Build history of the part. All positions in model axes, mm. Face numbers are marked on the shaded views. Give positions to 0.01 mm unless a question says otherwise; leave off trailing zeros. Order: outer loops, then holes, each group sorted by start corner. A loop starts at its lowest first (then second) coordinate and runs counter-clockwise, first axis right, second up. Notation, with made-up numbers: (10.25, 27) -> (22.25, 27) arc R14 cw to (22.25, 40) -> close; hole circle Ø11 at (15.5, -17). An arc over 180 degrees is marked (long way). One line per item, written item: value. Start each with the question number.
(1) Probe line 1 (X direction, y = 40, z = -12); line 2 (X direction, y = -5, z = 1); line 3 (Y direction, x = -14.5, z = -2.5). List the from-to ranges inside material, lowest first.
(2) Saw through at A-A on x = 0. Give the cut face in (y, z) (3 decimals), plus the area to 3 significant figures.
(3) Saw through at D-D on z = -11. Give the cut face in (x, y).
(4) Saw through at B-B on y = 0. Give the cut face in (x, z) (3 decimals), plus the area to 3 significant figures.
(5) Pin check, flat tips, straight feed: pin 1 (3.5 mm diameter, centred on x = -25, y = -1.5, fed in from +Z) (3 decimals); pin 2 (3.5 mm diameter, centred on x = -15, z = 0, fed in from +Y); pin 3 (23 mm diameter, centred on x = 0, y = 0, fed in from +Z). Stop position of each tip, or through.
(6) Saw through at C-C on x = -30. Give the cut face in (y, z) (3 decimals).
(7) Two-plate mould, pull along Y, no slides. Class the marked faces 1, 2 and 3: +Y half, -Y half, draft (parallel to the pull), parting line (faces both ways), or undercut.
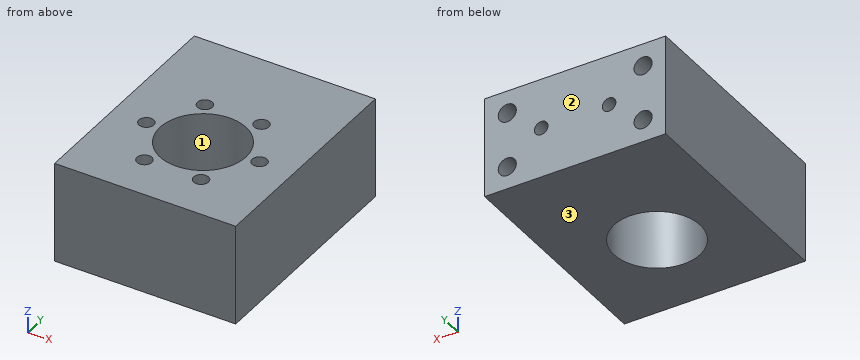
```python
from build123d import *

# Parameters (mm, degrees)
ESBO_O2_W                = 80
ESBO_O2_H                = 117.2
RESSALTO_EXTRUS_O2_DEPTH = 22.225
ESBO_O3_R                = 19
CORTE_EXTRUS_O1_DEPTH    = 45.45
ESBO_O4_R                = 3.3
CORTE_EXTRUS_O2_DEPTH    = 34.5
PADR_OCIRCULAR1_COUNT    = 6
ESBO_O10_R               = 4
ESBO_O10_R_2             = 3
CORTE_EXTRUS_O5_DEPTH    = 30
ESBO_O12_W               = 80
ESBO_O12_H               = 17.2
CORTE_EXTRUS_O7_DEPTH    = 45.45


with BuildPart() as part:
    # Esboço2 → Ressalto-extrusão2 (new body, symmetric)
    with BuildSketch(Plane.XY):
        Rectangle(ESBO_O2_W, ESBO_O2_H)
    extrude(amount=RESSALTO_EXTRUS_O2_DEPTH, both=True)

    # Esboço3 → Corte-extrusão1 (cut, through all)
    with BuildSketch(Plane.XY.offset(22.225)):
        Circle(ESBO_O3_R)
    extrude(amount=-CORTE_EXTRUS_O1_DEPTH, mode=Mode.SUBTRACT)

    # Esboço4 → Corte-extrusão2 (cut)
    with BuildSketch(Plane.XY.offset(22.225)):
        with Locations((12.5, 21.650635095)):
            Circle(ESBO_O4_R)
    corte_extrus_o2 = extrude(amount=-CORTE_EXTRUS_O2_DEPTH, mode=Mode.SUBTRACT)

    # PadrãoCircular1: Corte-extrusão2 ×6 about axis
    padr_ocircular1_axis = Axis((0, 0, 0), (0, 0, 1))
    for i in range(1, PADR_OCIRCULAR1_COUNT):
        add(corte_extrus_o2.rotate(padr_ocircular1_axis, i * 360 / PADR_OCIRCULAR1_COUNT), mode=Mode.SUBTRACT)

    # Esboço10 → Corte-extrusão5 (cut)
    with BuildSketch(Plane(origin=(0, 58.6, 0), x_dir=(1, 0, 0), z_dir=(0, 1, 0))):
        with Locations((-30, 12.225)):
            Circle(ESBO_O10_R)
        with Locations((30, 12.225)):
            Circle(ESBO_O10_R)
        with Locations((-30, -12.225)):
            Circle(ESBO_O10_R)
        with Locations((30, -12.225)):
            Circle(ESBO_O10_R)
        with Locations((-15, 0)):
            Circle(ESBO_O10_R_2)
        with Locations((15, 0)):
            Circle(ESBO_O10_R_2)
    extrude(amount=-CORTE_EXTRUS_O5_DEPTH, mode=Mode.SUBTRACT)

    # Esboço12 → Corte-extrusão7 (cut, through all)
    with BuildSketch(Plane.XY.offset(22.225)):
        with Locations((0, -50)):
            Rectangle(ESBO_O12_W, ESBO_O12_H)
    extrude(amount=-CORTE_EXTRUS_O7_DEPTH, mode=Mode.SUBTRACT)


solid = part.part
```
Results below:
1. line 1: x = -40 to -33.99, -26.01 to 26.01, 33.99 to 40
1. line 2: x = -40 to -18.33, 18.33 to 40
1. line 3: y = -41.4 to -24.28, -19.03 to -12.28, 12.28 to 19.03, 24.28 to 28.6
2. outline: (-41.4, -22.225) -> (-19, -22.225) -> (-19, 22.225) -> (-41.4, 22.225) -> close; (19, -22.225) -> (58.6, -22.225) -> (58.6, 22.225) -> (19, 22.225) -> close
2. area: 2,760 mm²
3. outline: (-40, -41.4) -> (40, -41.4) -> (40, 58.6) -> (33.81, 58.6) -> (33.81, 28.6) -> (26.19, 28.6) -> (26.19, 58.6) -> (-26.19, 58.6) -> (-26.19, 28.6) -> (-33.81, 28.6) -> (-33.81, 58.6) -> (-40, 58.6) -> close; hole circle Ø6.6 at (-25, 0); hole circle Ø38 at (0, 0); hole circle Ø6.6 at (-12.5, -21.65); hole circle Ø6.6 at (-12.5, 21.65); hole circle Ø6.6 at (12.5, -21.65); hole circle Ø6.6 at (12.5, 21.65); hole circle Ø6.6 at (25, 0)
4. outline: (-40, -22.225) -> (-19, -22.225) -> (-19, 22.225) -> (-21.7, 22.225) -> (-21.7, -12.275) -> (-28.3, -12.275) -> (-28.3, 22.225) -> (-40, 22.225) -> close; (19, -22.225) -> (40, -22.225) -> (40, 22.225) -> (28.3, 22.225) -> (28.3, -12.275) -> (21.7, -12.275) -> (21.7, 22.225) -> (19, 22.225) -> close
4. area: 1,410 mm²
5. pin 1: stops at z = -12.275
5. pin 2: stops at y = 28.6
5. pin 3: passes through
6. outline: (-41.4, -22.225) -> (58.6, -22.225) -> (58.6, -16.225) -> (28.6, -16.225) -> (28.6, -8.225) -> (58.6, -8.225) -> (58.6, 8.225) -> (28.6, 8.225) -> (28.6, 16.225) -> (58.6, 16.225) -> (58.6, 22.225) -> (-41.4, 22.225) -> close
7. face 1: undercut
7. face 2: +Y half
7. face 3: draft
